Verification items for the finished model (mm, model axes). Face numbers are marked on the shaded views. A direction names the side the tool comes from. Give positions to 0.01 mm unless a question says otherwise; leave off trailing zeros. Order: outer loops, then holes, each group sorted by start corner. A loop starts at its lowest first (then second) coordinate and runs counter-clockwise, first axis right, second up. Notation, with made-up numbers: (-35, -5.5) - (14, -5.5) arc R31 cw to (14, 26.5) - close; hole circle Ø2 at (87, 62.25). An arc over 180 degrees is marked (long way). Answer as a JSON object with one key per item and string values.
```python
from build123d import *
from OCP.BRepAlgoAPI import BRepAlgoAPI_Cut
from OCP.TopTools import TopTools_ListOfShape

# Parameters (mm, degrees)
SKIZZE1_R                       = 5.025
SKIZZE1_R_2                     = 2.75
AUFSATZ_LINEAR_AUSTRAGEN1_DEPTH = 10
AUFSATZ_LINEAR_AUSTRAGEN3_DEPTH = 10
SKIZZE4_W                       = 120
SKIZZE4_H                       = 15
AUFSATZ_LINEAR_AUSTRAGEN4_DEPTH = 80
AUFSATZ_LINEAR_AUSTRAGEN5_DEPTH = 10
AUFSATZ_LINEAR_AUSTRAGEN6_DEPTH = 10
VERRUNDUNG3_R                   = 10
VERRUNDUNG4_R                   = 5
VERRUNDUNG5_R                   = 10
SKIZZE11_R                      = 4.5
SCHNITT_LINEAR_AUSTRAGEN1_DEPTH = 3
VERRUNDUNG6_START               = 5.0000001
VERRUNDUNG6_DEPTH               = 4.9999999
VERRUNDUNG6_START_2             = -1e-07
VERRUNDUNG6_2_DEPTH             = 5.0000002
VERRUNDUNG6_START_3             = -67.945354479
VERRUNDUNG6_3_DEPTH             = 2.945354479
SKIZZE13_R                      = 5.05
SCHNITT_LINEAR_AUSTRAGEN3_DEPTH = 221.737400671
SKIZZE14_R                      = 13.3825
SCHNITT_LINEAR_AUSTRAGEN4_DEPTH = 5


with BuildPart() as part:
    # Skizze1 → Aufsatz-Linear austragen1 (new body)
    with BuildSketch(Plane.XY):
        with BuildLine():
            Line((90, 107.054645521), (-90, 107.054645521))
            ThreePointArc((-90, 107.054645521), (-97.071067812, 104.125713333), (-100, 97.054645521))
            Line((-100, 97.054645521), (-100, 77.054645521))
            ThreePointArc((-100, 77.054645521), (-97.071067812, 69.983577709), (-90, 67.054645521))
            Line((-90, 67.054645521), (-70, 67.054645521))
            ThreePointArc((-70, 67.054645521), (-59.393398282, 62.661247239), (-55, 52.054645521))
            Line((-55, 52.054645521), (-55, -67.945354479))
            Line((-55, -67.945354479), (-60, -67.945354479))
            Line((-60, -67.945354479), (-60, -82.945354479))
            Line((-60, -82.945354479), (60, -82.945354479))
            Line((60, -82.945354479), (60, -67.945354479))
            Line((60, -67.945354479), (55, -67.945354479))
            Line((55, -67.945354479), (55, 52.054645521))
            ThreePointArc((55, 52.054645521), (59.393398282, 62.661247239), (70, 67.054645521))
            Line((70, 67.054645521), (90, 67.054645521))
            ThreePointArc((90, 67.054645521), (97.071067812, 69.983577709), (100, 77.054645521))
            Line((100, 77.054645521), (100, 97.054645521))
            ThreePointArc((100, 97.054645521), (97.071067812, 104.125713333), (90, 107.054645521))
        make_face()
        with Locations((-70, 87.054645521)):
            Circle(SKIZZE1_R, mode=Mode.SUBTRACT)
        with Locations((-62.5, 94.554645521)):
            Circle(SKIZZE1_R_2, mode=Mode.SUBTRACT)
        with Locations((-77.5, 79.554645521)):
            Circle(SKIZZE1_R_2, mode=Mode.SUBTRACT)
        with Locations(Location((77.5, 79.554645521, 0), (0, 0, 180))):
            Circle(SKIZZE1_R_2, mode=Mode.SUBTRACT)
        with Locations(Location((62.5, 94.554645521, 0), (0, 0, 180))):
            Circle(SKIZZE1_R_2, mode=Mode.SUBTRACT)
        with Locations(Location((70, 87.054645521, 0), (0, 0, 180))):
            Circle(SKIZZE1_R, mode=Mode.SUBTRACT)
    extrude(amount=AUFSATZ_LINEAR_AUSTRAGEN1_DEPTH)

    # Skizze3 → Aufsatz-Linear austragen3 (add)
    with BuildSketch(Plane.XY.offset(10)):
        with BuildLine():
            Line((-72.845922337, 57.814606503), (-56.774282723, 37.352261221))
            add(Edge.make_bspline(
                [(-55, 18.961003518), (-46.636539725, 27.963101216), (-56.774282723, 37.352261221)],
                knots=[0, 0, 0, 1, 1, 1], degree=2))
            Line((-55, 18.961003518), (-43.333440031, 21.200490786))
            Line((-43.333440031, 21.200490786), (-45.498025685, 67.054645521))
            Line((-45.498025685, 67.054645521), (-90, 67.054645521))
            add(Edge.make_bspline(
                [(-90, 67.054645521), (-79.938268155, 65.656359823), (-72.845922337, 57.814606503)],
                knots=[0, 0, 0, 1, 1, 1], degree=2))
        make_face()
    extrude(amount=-AUFSATZ_LINEAR_AUSTRAGEN3_DEPTH)

    # Skizze4 → Aufsatz-Linear austragen4 (add)
    with BuildSketch(Plane.XY.offset(10)):
        with Locations((0, -75.445354479)):
            Rectangle(SKIZZE4_W, SKIZZE4_H)
    extrude(amount=AUFSATZ_LINEAR_AUSTRAGEN4_DEPTH)

    # Skizze9 → Aufsatz-Linear austragen5 (add)
    with BuildSketch(Plane.ZY.offset(51)):
        Polygon((10, 2.054645521), (80, -67.945354479), (6.644184354, -67.945354479), (6.644184354, 2.054645521), align=None)
    extrude(amount=-AUFSATZ_LINEAR_AUSTRAGEN5_DEPTH)

    # Skizze10 → Aufsatz-Linear austragen6 (add)
    with BuildSketch(Plane(origin=(51, 0, 0), x_dir=(0, 0, -1), z_dir=(1, 0, 0))):
        Polygon((-10, 2.204645521), (-80, -67.945354479), (-10, -67.945354479), align=None)
    extrude(amount=-AUFSATZ_LINEAR_AUSTRAGEN6_DEPTH)

    # Verrundung3
    verrundung3_edges = [part.edges().sort_by_distance(p)[0] for p in [
        (-46, -67.945354479, 80),
        (-46, 2.054645521, 10),
        (46, 2.204645521, 10),
        (46, -67.945354479, 80),
    ]]
    fillet(verrundung3_edges, radius=VERRUNDUNG3_R)

    # Verrundung4
    verrundung4_edges = [part.edges().sort_by_distance(p)[0] for p in [
        (-60, -75.445354479, 90),
        (60, -75.445354479, 90),
        (60, -75.445354479, 0),
        (-60, -75.445354479, 0),
    ]]
    fillet(verrundung4_edges, radius=VERRUNDUNG4_R)

    # Verrundung5
    # the kernel refuses this fillet: 10 mm, written as the material it adds along each edge
    with BuildSketch(Plane(origin=(-55, 35.554962551, 0), x_dir=(0, -1, 0), z_dir=(0, 0, 1))) as verrundung5_piece_1:
        with BuildLine():
            CenterArc((3.889315022, -10), VERRUNDUNG5_R, 90, 34.65693161)
            Line((-1.79729867, -1.774282723), (-1.911030943, -1.609768377))
            ThreePointArc((-1.911030943, -1.609768377), (-1.060157902, -0.723908397), (-0.133322184, 0.14908117))
            Line((-0.133322184, 0.14908117), (0, 0.2))
            Line((0, 0.2), (3.889315022, 0.2))
            Line((3.889315022, 0.2), (3.889315022, 0))
        make_face()
    extrude(amount=10)

    # Skizze11 → Schnitt-Linear austragen1 (cut)
    with BuildSketch(Plane.XY.offset(10)):
        with Locations((62.5, 94.554645521)):
            Circle(SKIZZE11_R)
        with Locations((77.5, 79.554645521)):
            Circle(SKIZZE11_R)
        with Locations((-62.5, 94.554645521)):
            Circle(SKIZZE11_R)
        with Locations((-77.5, 79.554645521)):
            Circle(SKIZZE11_R)
    extrude(amount=-SCHNITT_LINEAR_AUSTRAGEN1_DEPTH, mode=Mode.SUBTRACT)


with BuildPart() as verrundung6_tool:
    # Verrundung6: read off the stored shape, not the designer's step
    # Verrundung6 outline → Verrundung6 (new body)
    with BuildSketch(Plane.XY.offset(VERRUNDUNG6_START)):
        with BuildLine():
            Line((-57, -67.945354479), (-55, -67.945354479))
            Line((-55, -67.945354479), (-55, -65.945354479))
            ThreePointArc((-55, -65.945354479), (-55.585786438, -67.359568041), (-57, -67.945354479))
        make_face()
        with BuildLine():
            ThreePointArc((57, -67.945354479), (55.585786438, -67.359568041), (55, -65.945354479))
            Line((55, -65.945354479), (55, -67.945354479))
            Line((55, -67.945354479), (57, -67.945354479))
        make_face()
    extrude(amount=VERRUNDUNG6_DEPTH)


with BuildPart() as part_1:
    add(part.part)


with BuildPart() as part_2:
    # Verrundung6: joined with verrundung6_tool
    add(part_1.part.fuse(verrundung6_tool.part, tol=0.00001))


with BuildPart() as verrundung6_2_tool:
    # Verrundung6 2 outline → Verrundung6 2 (new body)
    with BuildSketch(Plane.XY.offset(VERRUNDUNG6_START_2)):
        with BuildLine():
            Line((-57, -67.945354479), (-55, -67.945354479))
            Line((-55, -67.945354479), (-55, -65.945354479))
            ThreePointArc((-55, -65.945354479), (-55.585786438, -67.359568041), (-57, -67.945354479))
        make_face()
        with BuildLine():
            ThreePointArc((57, -67.945354479), (55.585786438, -67.359568041), (55, -65.945354479))
            Line((55, -65.945354479), (55, -67.945354479))
            Line((55, -67.945354479), (57, -67.945354479))
        make_face()
    extrude(amount=VERRUNDUNG6_2_DEPTH)


with BuildPart() as part_3:
    add(part_2.part)


with BuildPart() as part_4:
    # Verrundung6 2: joined with verrundung6_2_tool
    add(part_3.part.fuse(verrundung6_2_tool.part, tol=0.00001))


with BuildPart() as verrundung6_3_tool:
    # Verrundung6 3 outline → Verrundung6 3 (new body)
    with BuildSketch(Plane(origin=(0, 0, 0), x_dir=(1, 0, 0), z_dir=(0, 1, 0)).offset(VERRUNDUNG6_START_3)):
        with BuildLine():
            Line((59, -3.288e-06), (55, 0))
            ThreePointArc((55, 0), (57.236067978, -0.527864045), (59, -2))
            Line((59, -2), (59, -3.288e-06))
        make_face()
        with BuildLine():
            ThreePointArc((-59, -2), (-57.236067913, -0.527864013), (-54.999999856, 0))
            Line((-54.999999856, 0), (-59, -5e-09))
            Line((-59, -5e-09), (-59, -2))
        make_face()
    extrude(amount=VERRUNDUNG6_3_DEPTH)


with BuildPart() as part_5:
    add(part_4.part)

    # Verrundung6 3: cut by verrundung6_3_tool, with a tolerance
    verrundung6_3_stock = TopTools_ListOfShape()
    verrundung6_3_stock.Append(part_5.part.wrapped)
    verrundung6_3_tools = TopTools_ListOfShape()
    verrundung6_3_tools.Append(verrundung6_3_tool.part.wrapped)
    verrundung6_3_cut = BRepAlgoAPI_Cut()
    verrundung6_3_cut.SetArguments(verrundung6_3_stock)
    verrundung6_3_cut.SetTools(verrundung6_3_tools)
    verrundung6_3_cut.SetFuzzyValue(0.00001)
    verrundung6_3_cut.Build()
    add(Compound.cast(verrundung6_3_cut.Shape()).solids(), mode=Mode.REPLACE)

    # Skizze13 → Schnitt-Linear austragen3 (cut, through all)
    with BuildSketch(Plane(origin=(0, -67.945354479, 0), x_dir=(1, 0, 0), z_dir=(0, 1, 0))):
        with Locations(Location((0, -37.5, 0), (0, 0, 270))):
            Circle(SKIZZE13_R)
    extrude(amount=-SCHNITT_LINEAR_AUSTRAGEN3_DEPTH, mode=Mode.SUBTRACT)

    # Skizze14 → Schnitt-Linear austragen4 (cut)
    with BuildSketch(Plane(origin=(0, -67.945354479, 0), x_dir=(1, 0, 0), z_dir=(0, 1, 0))):
        with Locations(Location((0, -37.5, 0), (0, 0, 270))):
            Circle(SKIZZE14_R)
    extrude(amount=-SCHNITT_LINEAR_AUSTRAGEN4_DEPTH, mode=Mode.SUBTRACT)


solid = part_5.part
```
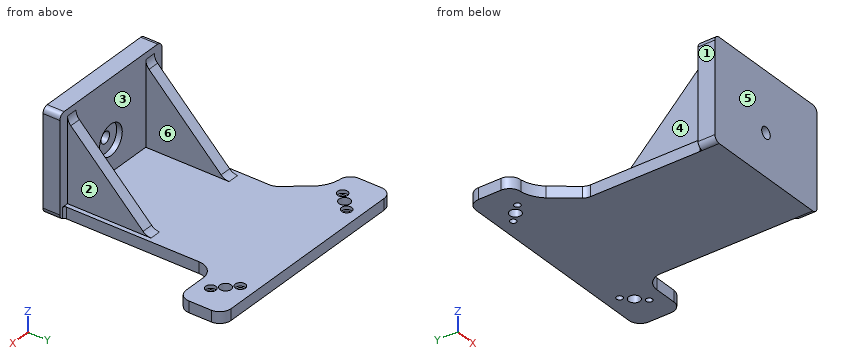
(1) Material ranges on line 1 along X through (y, z) = (-80.25, 37.5); line 2 along X through (y, z) = (-56, 10.5); line 3 along Z through (x, y) = (49.5, 92), recorded low to high. Write a range as [from, to].
Computed values:
{"line 1": "x = [-60, -5.05], [5.05, 60]", "line 2": "x = [-51, -41], [41, 51]", "line 3": "z = [0, 10]"}
(2) Release check for a two-part mould opening along X. For the marked faces 1, 2 and 3 record: pulls with the +X half, pulls with the -X half, needs draft (parallel to the pull), parting line crosses it, or undercut.
Computed values:
{"face 1": "pulls with the -X half", "face 2": "pulls with the +X half", "face 3": "undercut"}
(3) Section check C-C (x = -29). Record the cut outline in (y, z).
Computed values:
{"outline": "(-82.95, 0) - (107.05, 0) - (107.05, 10) - (-67.95, 10) - (-67.95, 90) - (-82.95, 90) - close"}
(4) Section check B-B (z = 36). Record the cut outline in (x, y), then the cut area to 3 significant figures.
Computed values:
{"outline": "(-60, -82.95) - (-4.82, -82.95) - (-4.82, -72.95) - (-13.3, -72.95) - (-13.3, -67.95) - (-41, -67.95) - (-41, -23.95) - (-51, -23.95) - (-51, -67.95) - (-60, -67.95) - close; (4.82, -82.95) - (60, -82.95) - (60, -67.95) - (51, -67.95) - (51, -23.85) - (41, -23.85) - (41, -67.95) - (13.3, -67.95) - (13.3, -72.95) - (4.82, -72.95) - close", "area": "2,450 mm²"}
(5) Gauge pin test, flat ends, axial feed: pin 1 Ø5 at (x, z) = (78, 3.5) entering from -Y; pin 2 Ø7 at (x, y) = (62, 95) entering from +Z; pin 3 Ø3 at (x, y) = (-4, 55.5) entering from +Z. Record the tip position at first contact, or that the pin passes through.
Computed values:
{"pin 1": "stops at y = 67.05", "pin 2": "stops at z = 7", "pin 3": "stops at z = 10"}
(6) Access from +Z, -Z, +X, -X, +Y, -Y to the whole of each face (thin tool, end or side, straight path). Record for the marked faces 4, 5 and 6.
Computed values:
{"face 4": "+Z, -X, +Y", "face 5": "+Z, -Z, +X, -X, -Y", "face 6": "+Z, +Y"}
(7) Section check D-D (y = 20). Record the cut outline in (x, z), then the cut area to 3 significant figures.
Computed values:
{"outline": "(-55, 0) - (55, 0) - (55, 10) - (-55, 10) - close", "area": "1,100 mm²"}
(8) Section check A-A (x = 0). Record the cut outline in (y, z).
Computed values:
{"outline": "(-82.95, 0) - (107.05, 0) - (107.05, 10) - (-67.95, 10) - (-67.95, 24.12) - (-72.95, 24.12) - (-72.95, 32.45) - (-82.95, 32.45) - close; (-82.95, 42.55) - (-72.95, 42.55) - (-72.95, 50.88) - (-67.95, 50.88) - (-67.95, 90) - (-82.95, 90) - close"}
